Can you work these out from the model? Positions are in its coordinate system, mm. A direction names the side the tool comes from. Coordinates: 2 decimals unless noted, no trailing zeros. Order: outer loops, then holes, each group sorted by start corner. A loop starts at its lowest first (then second) coordinate and runs counter-clockwise, first axis right, second up. Notation, with made-up numbers: (63, 28) -> (113, 28) arc R28 cw to (113, 61) -> close; hole circle Ø3 at (8, 54.5). An arc over 180 degrees is marked (long way). Answer as a JSON object with one key per item and string values. Group by question number.
(1) I want a section at D-D, the plane z = 0. List the corners of the cut face in (x, y) for me.
(2) I need wall thicknesses on line 1 (X direction, y = 14, z = 0); line 2 (Z direction, x = -37.5, y = 27.5); line 3 (Y direction, x = -44.5, z = 20.5). Which ranges of each line are inside material? Lowest first, please.
(3) If we mould it in two halves opening along Y, with no side actions, what happens to faces 1 (the flat face through (-55, 40, 0)), 2 (the flat face through (-30, 0, 0)), 3 (the flat face through (-55, 47, 20)), 4 (the flat face through (-7, 8, 7))? For each: pulls with the +Y half, pulls with the -Y half, needs draft (parallel to the pull), parting line crosses it, or undercut.
(4) I want a section at C-C, the plane x = -37.5. List the corners of the cut face in (y, z) for me, plus the area to 3 significant figures.
(5) I want a section at B-B, the plane y = 49. List the corners of the cut face in (x, z) for me.
(6) Which directions (+Z, -Z, +X, -X, +Y, -Y) give clear straight access to the entire face, cutting with the end or side of a thin tool? Please do faces 5 (the flat face through (-48, 10, 0)), 6 (the cylindrical face through (-55, 54, -18)), 7 (the flat face through (-12, 11, -12)).
(7) I want a section at A-A, the plane z = 10. List the corners of the cut face in (x, y) for me.
(8) For pin 1 (6 mm diameter, centred on x = -6, y = 9, fed in from -Z); pin 2 (6 mm diameter, centred on x = -5.5, y = 12, fed in from +Z); pin 3 (3 mm diameter, centred on x = -17.5, y = 19.5, fed in from -Z), each with a flat end and sliding along its axis, tell me the tip position at first contact or that it passes through.
from build123d import *

# Parameters (mm, degrees)
SKETCH2_W           = 10
SKETCH2_H           = 25
SKETCH2_W_2         = 23
SKETCH2_H_2         = 35
BOSS_EXTRUDE1_DEPTH = 25
SKETCH3_R           = 4
CUT_EXTRUDE2_DEPTH  = 61
CUT_EXTRUDE3_DEPTH  = 61
CUT_EXTRUDE4_DEPTH  = 61
CUT_EXTRUDE5_DEPTH  = 11
FILLET1_R           = 6


with BuildPart() as part:
    # Sketch2 → Boss-Extrude1 (new body, symmetric)
    with BuildSketch(Plane.XY):
        with Locations((-55, 47.5)):
            Rectangle(SKETCH2_W, SKETCH2_H)
        Polygon((-48, 20), (-48, 35), (-50, 35), (-60, 35), (-60, 20), align=None)
        with Locations((-36.5, 17.5)):
            Rectangle(SKETCH2_W_2, SKETCH2_H_2)
        Polygon((0, 10), (-25, 35), (-25, 0), (0, 0), align=None)
    extrude(amount=BOSS_EXTRUDE1_DEPTH, both=True)

    # Sketch3 → Cut-Extrude2 (cut, through all)
    with BuildSketch(Plane(origin=(0, 0, 0), x_dir=(1, 0, 0), z_dir=(0, 1, 0))):
        with Locations((-37.5, 0)):
            Circle(SKETCH3_R)
    extrude(amount=CUT_EXTRUDE2_DEPTH, mode=Mode.SUBTRACT)

    # Sketch3_5 → Cut-Extrude3 (cut, through all)
    with BuildSketch(Plane(origin=(0, 0, 0), x_dir=(1, 0, 0), z_dir=(0, 1, 0))):
        Polygon((0, 25), (-25, 25), (-12, 17.494446501), (0, 10.56624327), align=None)
        Polygon((-12, -17.494446501), (-25, -25), (0, -25), (0, -10.56624327), align=None)
    extrude(amount=CUT_EXTRUDE3_DEPTH, mode=Mode.SUBTRACT)

    # Sketch3_6 → Cut-Extrude4 (cut, through all)
    with BuildSketch(Plane(origin=(0, 0, 0), x_dir=(1, 0, 0), z_dir=(0, 1, 0))):
        Polygon((0, 10.56624327), (-12, 17.494446501), (-12, 7), (0, 7), align=None)
        Polygon((-12, -7), (-12, -17.494446501), (0, -10.56624327), (0, -7), align=None)
    extrude(amount=CUT_EXTRUDE4_DEPTH, mode=Mode.SUBTRACT)

    # Sketch6 → Cut-Extrude5 (cut, through all)
    with BuildSketch(Plane(origin=(-50, 0, 0), x_dir=(0, 0, -1), z_dir=(1, 0, 0))):
        with BuildLine():
            Line((-15, 55), (15, 55))
            ThreePointArc((15, 55), (18.535533906, 53.535533906), (20, 50))
            Line((20, 50), (20, 45))
            ThreePointArc((20, 45), (18.535533906, 41.464466094), (15, 40))
            Line((15, 40), (-15, 40))
            ThreePointArc((-15, 40), (-18.535533906, 41.464466094), (-20, 45))
            Line((-20, 45), (-20, 50))
            ThreePointArc((-20, 50), (-18.535533906, 53.535533906), (-15, 55))
        make_face()
    extrude(amount=-CUT_EXTRUDE5_DEPTH, mode=Mode.SUBTRACT)

    # Fillet1
    fillet1_edges = [part.edges().sort_by_distance(p)[0] for p in [
        (-55, 60, -25),
        (-55, 60, 25),
    ]]
    fillet(fillet1_edges, radius=FILLET1_R)


solid = part.part
Computed values:
{
 "1": {"outline": "(-60, 20) -> (-48, 20) -> (-48, 0) -> (-41.5, 0) -> (-41.5, 35) -> (-50, 35) -> (-50, 40) -> (-60, 40) -> close; (-60, 55) -> (-50, 55) -> (-50, 60) -> (-60, 60) -> close; (-33.5, 0) -> (0, 0) -> (0, 10) -> (-25, 35) -> (-33.5, 35) -> close"},
 "2": {"line 1": "x = -48 to -41.5, -33.5 to -4", "line 2": "z = -25 to -4, 4 to 25", "line 3": "y = 0 to 35"},
 "3": {"face 1": "undercut", "face 2": "pulls with the -Y half", "face 3": "undercut", "face 4": "needs draft"},
 "4": {"outline": "(0, -25) -> (35, -25) -> (35, -4) -> (0, -4) -> close; (0, 4) -> (35, 4) -> (35, 25) -> (0, 25) -> close", "area": "1,470 mm2"},
 "5": {"outline": "(-60, -25) -> (-50, -25) -> (-50, -20) -> (-60, -20) -> close; (-60, 20) -> (-50, 20) -> (-50, 25) -> (-60, 25) -> close"},
 "6": {"face 5": "+Z, -Z, -X, -Y", "face 6": "+X, -X", "face 7": "-Z, +X, +Y, -Y"},
 "7": {"outline": "(-60, 20) -> (-48, 20) -> (-48, 0) -> (-12, 0) -> (-12, 22) -> (-25, 35) -> (-50, 35) -> (-50, 40) -> (-60, 40) -> close; (-60, 55) -> (-50, 55) -> (-50, 60) -> (-60, 60) -> close"},
 "8": {"pin 1": "stops at z = -7", "pin 2": "stops at z = 7", "pin 3": "stops at z = -21.54"}
}
